Source: CAD feature listing. Evaluate the final solid. Frame: model axes, mm. A direction names the side the tool comes from. Round coordinates to 2 decimals unless told otherwise and drop trailing zeros. Order: outer loops, then holes, each group sorted by start corner. A loop starts at its lowest first (then second) coordinate and runs counter-clockwise, first axis right, second up. Notation, with made-up numbers: (6.5, 89.25) - (57.5, 89.25) arc R23 ccw to (57.5, 125.25) - close; hole circle Ø9 at (56.5, 14.5). An arc over 180 degrees is marked (long way). Return JSON: item names as keys, results as strings. Group by question number.
1) Contact query for flat-ended pins moving along their axis: P1, Ø4, axis at x = 34, y = 18.5, coming from the -Z side; P2, Ø5, axis at x = 25, z = 21, coming from the -Y side; P3, Ø1.5, axis at x = 14.5, y = -16, coming from the +Z side; P4, Ø2.5, axis at x = 42.84, y = 8.25, coming from the +Z side. Output: stop coordinate, or through.
2) Section D-D, the plane x = 43. Return loops of the section in (y, z).
3) Section C-C, the plane z = 24.75. Return loops of the section in (x, y).
4) Section B-B, the plane x = 15. Return loops of the section in (y, z).
5) Ray query, line 1 (Y direction, x = 16, z = 19); line 2 (X direction, y = 23, z = 15); line 3 (Y direction, x = 24.5, z = 26.25). Return the intervals inside material, ascending. Write a range as from..to.
6) Access query for faces 1 (the flat face through (31, 14, 18)), 2 (the flat face through (36.33, 19.92, 13.4)), 3 (the flat face through (16, -30.75, 15)), 4 (the flat face through (22, -35, 15)), 5 (the flat face through (33, 20, 18.25)). Directions: +Z, -Z, +X, -X, +Y, -Y. A direction counts if a zero-diameter tool reaches every point of the face in a straight line with its end or side. Return the directions, or none.
7) Mould query, pull axis Z, two halves, no side actions, for faces 6 (the cylindrical face through (15.81, -29.04, 9.25)), 7 (the flat face through (30.7, 19.92, 13.35)), 8 (the flat face through (36.3, 19.92, 16.65)). Classes: pulls with the +Z half, pulls with the -Z half, needs draft (parallel to the pull), parting line crosses it, or undercut.
8) Section A-A, the plane x = 3.5. Return loops of the section in (y, z).
```python
from build123d import *

# Parameters (mm, degrees)
SKETCH_1_W          = 47
SKETCH_1_H          = 30
EXTRUDE_1_DEPTH     = 11
SKETCH_2_R          = 6
EXTRUDE_2_DEPTH     = 3
EXTRUDE_3_DEPTH     = 12
SKETCH_4_R          = 14
EXTRUDE_4_DEPTH     = 35
SKETCH_5_R          = 5
EXTRUDE_5_DEPTH     = 2
SKETCH_6_R          = 1.5
CUT_EXTRUDE_1_DEPTH = 67.917860097
CUT_EXTRUDE_2_DEPTH = 67.917860097
SKETCH_9_R          = 1.5
CUT_EXTRUDE_3_DEPTH = 8


with BuildPart() as part:
    # 草图1 → 凸台-拉伸1 (new body)
    with BuildSketch(Plane(origin=(0, 0, 0), x_dir=(1, 0, 0), z_dir=(0, 1, 0))):
        with Locations((23.5, -15)):
            Rectangle(SKETCH_1_W, SKETCH_1_H)
    extrude(amount=EXTRUDE_1_DEPTH)

    # 草图2 → 凸台-拉伸2 (add)
    with BuildSketch(Plane(origin=(0, 11, 0), x_dir=(1, 0, 0), z_dir=(0, 1, 0))):
        with Locations(Location((33.5, -15, 0), (0, 0, 270))):
            Circle(SKETCH_2_R)
    extrude(amount=EXTRUDE_2_DEPTH)

    # 草图3 → 凸台-拉伸3 (add)
    with BuildSketch(Plane(origin=(0, 14, 0), x_dir=(1, 0, 0), z_dir=(0, 1, 0))):
        Polygon((37.25277675, -15), (35.376388375, -11.75), (31.623611625, -11.75), (29.74722325, -15), (31.623611625, -18.25), (35.376388375, -18.25), align=None)
    extrude(amount=EXTRUDE_3_DEPTH)

    # 草图4 → 凸台-拉伸4 (add)
    with BuildSketch(Plane.XZ):
        with Locations(Location((16, 15, 0), (0, 0, 90))):
            Circle(SKETCH_4_R)
    extrude(amount=EXTRUDE_4_DEPTH)

    # 草图5 → 凸台-拉伸5 (add)
    with BuildSketch(Plane.XZ.offset(35)):
        with Locations(Location((16, 15, 0), (0, 0, 270))):
            Circle(SKETCH_5_R)
    extrude(amount=EXTRUDE_5_DEPTH)

    # 草图6 → 切除-拉伸1 (cut, through all)
    with BuildSketch(Plane.XY.offset(30)):
        with Locations((3.340757383, 8.25)):
            Circle(SKETCH_6_R)
        with Locations((32.340757383, 8.25)):
            Circle(SKETCH_6_R)
        with Locations((42.840757383, 8.25)):
            Circle(SKETCH_6_R)
    extrude(amount=-CUT_EXTRUDE_1_DEPTH, mode=Mode.SUBTRACT)

    # 草图7 → 切除-拉伸2 (cut, through all)
    with BuildSketch(Plane.ZY):
        with BuildLine():
            Line((11, -27.25), (19, -27.25))
            ThreePointArc((19, -27.25), (20.75, -29), (19, -30.75))
            Line((19, -30.75), (11, -30.75))
            ThreePointArc((11, -30.75), (9.25, -29), (11, -27.25))
        make_face()
    extrude(amount=-CUT_EXTRUDE_2_DEPTH, mode=Mode.SUBTRACT)

    # 草图9 → 切除-拉伸3 (cut)
    with BuildSketch(Plane(origin=(0, 26, 0), x_dir=(1, 0, 0), z_dir=(0, 1, 0))):
        with Locations(Location((33.5, -15, 0), (0, 0, 270))):
            Circle(SKETCH_9_R)
    extrude(amount=-CUT_EXTRUDE_3_DEPTH, mode=Mode.SUBTRACT)


solid = part.part
```
Geometry check:
{
 "1": {"P1": "z = 11.75", "P2": "y = -35", "P3": "z = 28.98", "P4": "through"},
 "2": {"outline": "(0, 0) - (6.76, 0) - (6.76, 30) - (0, 30) - close; (9.74, 0) - (11, 0) - (11, 30) - (9.74, 30) - close"},
 "3": {"outline": "(0, 0) - (5.95, 0) - (5.95, -35) - (26.05, -35) - (26.05, 0) - (47, 0) - (47, 11) - (0, 11) - close; hole circle Ø3 at (3.34, 8.25); hole circle Ø3 at (32.34, 8.25); hole circle Ø3 at (42.84, 8.25)"},
 "4": {"outline": "(-37, 10.1) - (-35, 10.1) - (-35, 1.04) - (0, 1.04) - (0, 0) - (11, 0) - (11, 30) - (0, 30) - (0, 28.96) - (-35, 28.96) - (-35, 19.9) - (-37, 19.9) - close; hole (-30.75, 11) arc R1.75 ccw to (-27.25, 11) - (-27.25, 19) arc R1.75 ccw to (-30.75, 19) - close"},
 "5": {"line 1": "-37..-30.75, -27.25..11", "line 2": "29.75..32, 35..37.25", "line 3": "0..11"},
 "6": {"face 1": "+Y", "face 2": "-Z, +X, +Y", "face 3": "+X, -X", "face 4": "-Y", "face 5": "+Z, +X, -X, +Y"},
 "7": {"face 6": "undercut", "face 7": "pulls with the -Z half", "face 8": "pulls with the +Z half"},
 "8": {"outline": "(-35, 8.7) - (0, 8.7) - (0, 0) - (6.76, 0) - (6.76, 30) - (0, 30) - (0, 21.3) - (-35, 21.3) - close; (9.74, 0) - (11, 0) - (11, 30) - (9.74, 30) - close; hole (-30.75, 11) arc R1.75 ccw to (-27.25, 11) - (-27.25, 19) arc R1.75 ccw to (-30.75, 19) - close"}
}
